Design review of the part shown in the three views and the two pictorial views. Dimensions are in mm from the part's minimum x, y and z. A direction names the side the tool comes from. Round coordinates to 2 decimals unless told otherwise and drop trailing zeros. Write each loop counter-clockwise with the first axis right and the second up, starting at its lowest first coordinate (ties: lowest second). Pieces come first, ordered by that corner, then holes. Notation, with made-up numbers: (3.25, -19.5) - (13.25, -19.5) arc R26 ccw to (13.25, -1.5) - close; hole circle Ø4 at (52, 69). An arc over 180 degrees is marked (long way). Use one line per item in the form item = value.
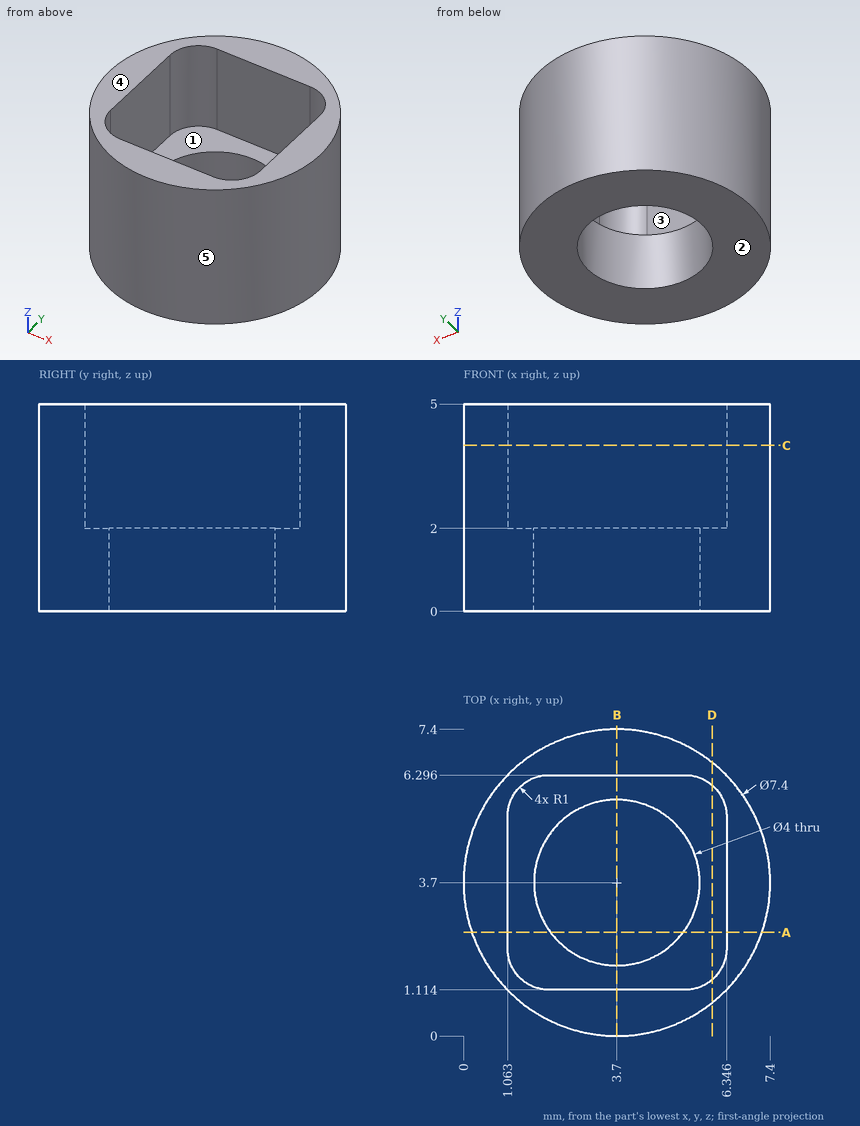
Q1. We need section A-A on y = 2.5. Write out the cut boundary in (x, z).
Calculated:
outline = (0.2, 0) - (2.1, 0) - (2.1, 2) - (1.06, 2) - (1.06, 5) - (0.2, 5) - close; (5.3, 0) - (7.2, 0) - (7.2, 5) - (6.35, 5) - (6.35, 2) - (5.3, 2) - close
Q2. Machinability: for the marked faces 1 and 2, which of the approach directions +Z, -Z, +X, -X, +Y, -Y give a long, thin tool a straight path to every point of the face, cutting with its end or side? Answer none if there is none.
Calculated:
face_1 = +Z
face_2 = -Z, +X, -X, +Y, -Y
Q3. For P1, Ø1, axis at y = 4.5, z = 2, coming from the +X side; P2, Ø1.5, axis at x = 4, z = 4, coming from the -Y side; P3, Ø2.5, axis at x = 3.5, y = 3.5, coming from the +Z side, all flat-tipped, find the tip position at first contact; note any pin that passes through.
Calculated:
P1 = 7.39
P2 = 0
P3 = through
Q4. We need section D-D on x = 6. Write out the cut boundary in (y, z).
Calculated:
outline = (0.8, 0) - (6.6, 0) - (6.6, 5) - (6.05, 5) - (6.05, 2) - (1.36, 2) - (1.36, 5) - (0.8, 5) - close
Q5. We need section B-B on x = 3.7. Write out the cut boundary in (y, z) (1 decimal).
Calculated:
outline = (0, 0) - (1.7, 0) - (1.7, 2) - (1.1, 2) - (1.1, 5) - (0, 5) - close; (5.7, 0) - (7.4, 0) - (7.4, 5) - (6.3, 5) - (6.3, 2) - (5.7, 2) - close
Q6. To check wall thickness, follow line 1 along Y through (x, z) = (3.7, 0.75); line 2 along X through (y, z) = (6, 3.5) (1 decimal); line 3 along X through (y, z) = (2.25, 3.4) (1 decimal). State the ranges of each line that lie inside material, in increasing order. Write a range as from..to.
Calculated:
line_1 = 0..1.7, 5.7..7.4
line_2 = 0.8..1.4, 6.1..6.6
line_3 = 0.3..1.1, 6.3..7.1
Q7. Draft analysis for pull direction X (two halves, no side actions). For the marked faces 3, 4 and 5, state which applies: released by +X, released by -X, zero draft, split by the parting line, or undercut.
Calculated:
face_3 = undercut
face_4 = zero draft
face_5 = split by the parting line
Q8. We need section C-C on z = 4. Write out the cut boundary in (x, y) (1 decimal).
Calculated:
outline = circle Ø7.4 at (3.7, 3.7); hole (1.1, 2.1) arc R1 ccw to (2.1, 1.1) - (5.3, 1.1) arc R1 ccw to (6.3, 2.1) - (6.3, 5.3) arc R1 ccw to (5.3, 6.3) - (2.1, 6.3) arc R1 ccw to (1.1, 5.3) - close
